Design review of the part built by this model. Coordinates are the model's own, in mm. Give positions to 0.01 mm unless a question says otherwise; leave off trailing zeros. Write each loop counter-clockwise with the first axis right and the second up, starting at its lowest first coordinate (ties: lowest second). Pieces come first, ordered by that corner, then holes. Notation, with made-up numbers: M 38,87 L 71,87 A18 ccw 71,111 Z; hole C 15.5,29 d7. An arc over 180 degrees is marked long. Answer in a Markdown table with one row per item.
```python
from build123d import *
from build123d.topology import SkipClean

# Parameters (mm, degrees)
SKETCH_1_R          = 55
EXTRUDE_1_DEPTH     = 4
SKETCH_4_R          = 15
SKETCH_3_R          = 15
SKETCH_7_R          = 15
SKETCH_6_R          = 15
SKETCH_9_R          = 5
CUT_EXTRUDE_1_DEPTH = 24
CHAMFER_1_SIZE      = 5
CHAMFER_2_SIZE      = 4


with BuildPart() as part:
    # 草图1 → 凸台-拉伸1 (new body)
    with BuildSketch(Plane(origin=(0, 0, 0), x_dir=(0, 0, -1), z_dir=(1, 0, 0))):
        Circle(SKETCH_1_R)
        with BuildLine():
            Line((-3, 39.115214431), (-3, 19.899748742))
            ThreePointArc((-3, 19.899748742), (-4.077383711, 16.026765396), (-7, 13.266499161))
            ThreePointArc((-7, 13.266499161), (-12.990381057, 7.5), (-14.989125293, -0.571071754))
            ThreePointArc((-14.989125293, -0.571071754), (-15.918277829, -4.482264824), (-18.73368794, -7.35179816))
            Line((-18.73368794, -7.35179816), (-35.374769372, -16.959531004))
            ThreePointArc((-35.374769372, -16.959531004), (-41.996474081, -17.39278273), (-46.370097033, -12.402181305))
            ThreePointArc((-46.370097033, -12.402181305), (-41.569219382, 24), (-12.444444444, 46.358772659))
            ThreePointArc((-12.444444444, 46.358772659), (-5.935645354, 45.066404788), (-3, 39.115214431))
        make_face(mode=Mode.SUBTRACT)
        with BuildLine():
            Line((3, 39.115214431), (3, 19.899748742))
            ThreePointArc((3, 19.899748742), (4.077383711, 16.026765396), (7, 13.266499161))
            ThreePointArc((7, 13.266499161), (12.990381057, 7.5), (14.989125293, -0.571071754))
            ThreePointArc((14.989125293, -0.571071754), (15.918277829, -4.482264824), (18.73368794, -7.35179816))
            Line((18.73368794, -7.35179816), (35.374769372, -16.959531004))
            ThreePointArc((35.374769372, -16.959531004), (41.996474081, -17.39278273), (46.370097033, -12.402181305))
            ThreePointArc((46.370097033, -12.402181305), (41.569219382, 24), (12.444444444, 46.358772659))
            ThreePointArc((12.444444444, 46.358772659), (5.935645354, 45.066404788), (3, 39.115214431))
        make_face(mode=Mode.SUBTRACT)
        with BuildLine():
            Line((32.374769372, -22.155683427), (15.73368794, -12.547950582))
            ThreePointArc((15.73368794, -12.547950582), (11.840894118, -11.544500572), (7.989125293, -12.695427407))
            ThreePointArc((7.989125293, -12.695427407), (0, -15), (-7.989125293, -12.695427407))
            ThreePointArc((-7.989125293, -12.695427407), (-11.840894118, -11.544500572), (-15.73368794, -12.547950582))
            Line((-15.73368794, -12.547950582), (-32.374769372, -22.155683427))
            ThreePointArc((-32.374769372, -22.155683427), (-36.060828727, -27.673622059), (-33.925652589, -33.956591354))
            ThreePointArc((-33.925652589, -33.956591354), (0, -48), (33.925652589, -33.956591354))
            ThreePointArc((33.925652589, -33.956591354), (36.060828727, -27.673622059), (32.374769372, -22.155683427))
        make_face(mode=Mode.SUBTRACT)
    extrude(amount=EXTRUDE_1_DEPTH)

    # 草图4 → 放样1 section 0
    with BuildSketch(Plane.ZY):
        Circle(SKETCH_4_R)
    # 草图3 → 放样1 section 1
    with BuildSketch(Plane.ZY.offset(6)):
        Circle(SKETCH_3_R)
    loft()

    # 草图7 → 放样2 section 0
    with SkipClean():  # the faces are left unmerged after this step: merging them gives an invalid solid
        with BuildSketch(Plane(origin=(10, 0, 0), x_dir=(0, 0, -1), z_dir=(1, 0, 0))):
            Circle(SKETCH_7_R)
        # 草图6 → 放样2 section 1
        with BuildSketch(Plane(origin=(4, 0, 0), x_dir=(0, 0, -1), z_dir=(1, 0, 0))):
            Circle(SKETCH_6_R)
        loft()

    # 草图9 → 切除-拉伸1 (cut, symmetric)
    with SkipClean():  # the faces are left unmerged after this step: merging them gives an invalid solid
        with BuildSketch(Plane.ZY.offset(6)):
            Circle(SKETCH_9_R)
        extrude(amount=CUT_EXTRUDE_1_DEPTH, both=True, mode=Mode.SUBTRACT)

    # 倒角1
    chamfer_1_edges = [part.edges().sort_by_distance(p)[0] for p in [
        (10, 0, 15),
    ]]
    chamfer(chamfer_1_edges, length=CHAMFER_1_SIZE)

    # 倒角2
    chamfer_2_edges = [part.edges().sort_by_distance(p)[0] for p in [
        (-6, 0, -15),
    ]]
    chamfer(chamfer_2_edges, length=CHAMFER_2_SIZE)


solid = part.part
```
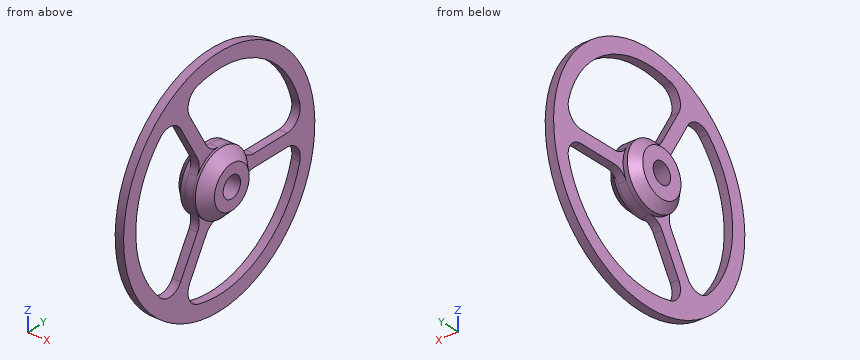
1) Add section D-D (y = 34.5). Write out the cut boundary in (x, z), and give its area (3 significant figures).
Geometry says:
| item | result |
|---|---|
| outline | M 0,-42.83 L 4,-42.83 L 4,-33.37 L 0,-33.37 Z; M 0,-3 L 4,-3 L 4,3 L 0,3 Z; M 0,33.37 L 4,33.37 L 4,42.83 L 0,42.83 Z |
| area | 99.7 mm^2 |
2) Add section B-B (y = -40.5). Write out the cut boundary in (x, z).
Geometry says:
| item | result |
|---|---|
| outline | M 0,-37.21 L 4,-37.21 L 4,-25.76 L 0,-25.76 Z; M 0,25.76 L 4,25.76 L 4,37.21 L 0,37.21 Z |
3) Add section C-C (x = 8.25). Write out the cut boundary in (y, z).
Geometry says:
| item | result |
|---|---|
| outline | C 0,0 d23.5; hole C 0,0 d10 |
4) Insertion check: P1, Ø8, axis at y = -21, z = 6, coming from the -X side; P2, Ø6, axis at x = 1, y = -20.5, coming from the +Z side; P3, Ø3, axis at x = 3, y = 31.5, coming from the +Z side; P4, Ø1, axis at x = 1.5, z = -26, coming from the +Y side. Each pin has a flat end and moves straight along its axis. Give the tip position at first contact, or say it passes through.
Geometry says:
| item | result |
|---|---|
| P1 | through |
| P2 | z = 52.14 |
| P3 | z = 46.1 |
| P4 | y = 48.73 |
5) Add section A-A (z = 0). Write out the cut boundary in (x, y), and give its area (3 significant figures).
Geometry says:
| item | result |
|---|---|
| outline | M -6,-11 L -2,-15 L 5,-15 L 10,-10 L 10,-5 L -6,-5 Z; M -6,5 L 10,5 L 10,10 L 5,15 L 4,15 L 4,55 L 0,55 L 0,15 L -2,15 L -6,11 Z; M 0,-55 L 4,-55 L 4,-48 L 0,-48 Z |
| area | 467 mm^2 |
6) To check wall thickness, follow probe 1 along Y at (x, z) = (3.5, 0); probe 2 along Y at (x, z) = (4.75, 0); probe 3 along Z at (x, y) = (2.5, 17.5). State the ranges of each line that lie inside material, in increasing order. Write a range as [from, to].
Geometry says:
| item | result |
|---|---|
| probe 1 | [-55, -48], [-15, -5], [5, 55] |
| probe 2 | [-15, -5], [5, 15] |
| probe 3 | [-52.14, -44.7], [-3.39, 3.39], [44.7, 52.14] |
